from build123d import *

# Parameters (mm, degrees)
SKETCH1_R          = 12.7
EXTRUDE1_DEPTH     = 7.9375
CHAMFER1_SIZE      = 1.360714286
CHAMFER2_SIZE      = 0.907142857
CUT_SWEEP1_PITCH   = 1.814285714
CUT_EXTRUDE1_DEPTH = 20.636290712


with BuildPart() as part:
    # Sketch1 → Extrude1 (new body)
    with BuildSketch(Plane(origin=(0, 0, 0), x_dir=(1, 0, 0), z_dir=(0, 1, 0))):
        with Locations(Location((0, 0, 0), (0, 0, 270))):
            Circle(SKETCH1_R)
    extrude(amount=-EXTRUDE1_DEPTH)

    # Chamfer1
    chamfer1_edges = [part.edges().sort_by_distance(p)[0] for p in [
        (0, -7.9375, -12.7),
    ]]
    chamfer(chamfer1_edges, length=CHAMFER1_SIZE)

    # Chamfer2
    chamfer2_edges = [part.edges().sort_by_distance(p)[0] for p in [
        (0, 0, -12.7),
    ]]
    chamfer(chamfer2_edges, length=CHAMFER2_SIZE)

    # Cut-Sweep1: the profile of Sketch3 profile screwed along a right-hand helix of 5.375 turns, 6 arcs to a turn; built about Z, then put on its axis
    cut_sweep1_z = Axis((0, 0, 0), (0, 0, 1))
    cut_sweep1_corners = [(12.7003, 0, 0.000173205), (11.521586861, 0, -0.680357143), (11.521586861, 0, -0.907142857), (12.7003, 0, -1.587673205)]
    with BuildLine(mode=Mode.PRIVATE) as cut_sweep1_profile:
        Line(cut_sweep1_corners[0], cut_sweep1_corners[1])
        Line(cut_sweep1_corners[1], cut_sweep1_corners[2])
        Line(cut_sweep1_corners[2], cut_sweep1_corners[3])
        Line(cut_sweep1_corners[3], cut_sweep1_corners[0])
    cut_sweep1_cap = Face(cut_sweep1_profile.wire())
    cut_sweep1_turn_angles = [0, 30, 60, 90, 120, 150, 180, 210, 240, 270, 300, 330, 360]
    cut_sweep1_turn_weights = [1, 0.8660254037844387, 1, 0.8660254037844387, 1, 0.8660254037844387, 1, 0.8660254037844387, 1, 0.8660254037844387, 1, 0.8660254037844387, 1]
    cut_sweep1_turn_rails = [Edge.make_bspline([Vector(p[0], p[1], 0).rotate(cut_sweep1_z, cut_sweep1_turn_angles[k]) / cut_sweep1_turn_weights[k] + Vector(0, 0, p[2] + CUT_SWEEP1_PITCH * cut_sweep1_turn_angles[k] / 360) for k in range(13)], [0, 0, 0, 1, 1, 2, 2, 3, 3, 4, 4, 5, 5, 6, 6, 6], 2, cut_sweep1_turn_weights) for p in cut_sweep1_corners]
    cut_sweep1_turn_sides = [Face.make_surface_from_curves(cut_sweep1_turn_rails[p[0]], cut_sweep1_turn_rails[p[1]]) for p in [(0, 1), (1, 2), (2, 3), (3, 0)]]
    cut_sweep1_last_angles = [1800, 1830, 1860, 1890, 1920, 1927.5, 1935]
    cut_sweep1_last_weights = [1, 0.8660254037844387, 1, 0.8660254037844387, 1, 0.991444861373807, 1]
    cut_sweep1_last_rails = [Edge.make_bspline([Vector(p[0], p[1], 0).rotate(cut_sweep1_z, cut_sweep1_last_angles[k]) / cut_sweep1_last_weights[k] + Vector(0, 0, p[2] + CUT_SWEEP1_PITCH * cut_sweep1_last_angles[k] / 360) for k in range(7)], [0, 0, 0, 1, 1, 2, 2, 3, 3, 3], 2, cut_sweep1_last_weights) for p in cut_sweep1_corners]
    cut_sweep1_last_sides = [Face.make_surface_from_curves(cut_sweep1_last_rails[p[0]], cut_sweep1_last_rails[p[1]]) for p in [(0, 1), (1, 2), (2, 3), (3, 0)]]
    cut_sweep1 = Plane(origin=(0, 0, 0), x_dir=(0, 0, 1), z_dir=(0, -1, 0)) * Solid(Shell([*[p.moved(Location((0, 0, CUT_SWEEP1_PITCH * i))) for i in range(5) for p in cut_sweep1_turn_sides], *cut_sweep1_last_sides, cut_sweep1_cap, cut_sweep1_cap.rotate(cut_sweep1_z, 1935).moved(Location((0, 0, CUT_SWEEP1_PITCH * 1935 / 360)))]))
    add(cut_sweep1, mode=Mode.SUBTRACT)

    # Sketch4 → Cut-Extrude1 (cut, through all)
    with BuildSketch(Plane(origin=(0, 0, 0), x_dir=(1, 0, 0), z_dir=(0, 1, 0))):
        Polygon((0, 3.666174209), (-3.175, 1.833087105), (-3.175, -1.833087105), (0, -3.666174209), (3.175, -1.833087105), (3.175, 1.833087105), align=None)
    extrude(amount=-CUT_EXTRUDE1_DEPTH, mode=Mode.SUBTRACT)


solid = part.part
Check sheet for the modelled part. Datum: model origin and axes. Units: mm. A direction names the side the tool comes from. Round coordinates to 2 decimals unless told otherwise and drop trailing zeros.
1. Gauge pin test, flat end, axial feed: pin 1 Ø3 at (y, z) = (-3, -5) entering from -X. Record the tip position at first contact, or that the pin passes through.
2. Scan lines: probe 1 along Y at (x, z) = (4.5, 10.75); probe 2 along Z at (x, y) = (1.5, -3); probe 3 along Z at (x, y) = (1.25, -0.5). Record each from-to range of solid material in increasing order.
3. Set-up check for faces 4 (the flat face through (-1.61, -3.913, 2.737)), 5 (the flat face through (2.7, -7.938, 2.4)): record each of +Z, -Z, +X, -X, +Y, -Y from which the full face is reachable in a straight line by a thin tool's end or side.
4. Mould release check, pull along X, two halves, no side actions. Record for faces 1 (the conical face through (3.471, -7.72, 11.023)), 2 (the flat face through (-2, 0, 3)), 3 (the flat face through (-1.57, -3.91, -2.76)): released by +X, released by -X, zero draft, split by the parting line, or undercut.
Recorded:
1. pin 1: stops at x = -12.19
2. probe 1: y = -7.62 to -6.54, -6.16 to -4.73, -4.35 to -2.91, -2.53 to -1.1, -0.72 to 0
2. probe 2: z = -12.58 to -2.8, 2.8 to 11.57
2. probe 3: z = -11.88 to -2.94, 2.94 to 12.11
3. face 4: +Y, -Y
3. face 5: +Z, -Z, +X, -X, -Y
4. face 1: split by the parting line
4. face 2: zero draft
4. face 3: undercut
